from build123d import *

# Parameters (mm, degrees)
F0_W     = 87
F0_H     = 2
F0_W_2   = 29
F1_DEPTH = 2


# Not quite as in the source:
# - ends of sketch curves that miss each other by under 0.0002 mm in the source are joined


with BuildPart() as f1:
    # F0 (on Front) → F1 (new body)
    with BuildSketch(Plane.XZ):
        Polygon((-74.1755201817, -53.7046223087), (-74.1755201817, -54.8843706005), (16.8244798183, -54.8843706005), (16.8244798183, -52.8843706005), (-12.1755201817, -52.8843706005), (-12.1755201817, -50.8843706005), (16.8244798183, -50.8843706005), (16.8244798183, -44.8844749875), (-12.1755201817, -44.8844749875), (-12.1755201817, -42.8844749875), (16.8244798183, -42.8844749875), (16.8244798183, -36.7078750432), (-12.1755201817, -36.7078750432), (-12.1754285991, -34.7078750432), (16.8244798183, -34.7078750432), (16.8244798183, -28.7078750432), (-12.1755201817, -28.7078750432), (-12.1754285991, -26.7078750432), (16.8244798183, -26.7078750432), (16.8244798183, -20.5312750988), (-12.1755201817, -20.5312750988), (-12.1755201817, -18.5312750988), (16.8244798183, -18.5312750988), (16.8244798183, -12.5313794858), (-12.1755201817, -12.5313794858), (-12.1755201817, -10.5313794858), (16.8244798183, -10.5313794858), (16.8244798183, -4.5313794858), (-12.1755201817, -4.5313794858), (-12.1755201817, -2.5313794858), (16.8244798183, -2.5313794858), (16.8244798183, 3.4685161272), (-12.1755201817, 3.4685161272), (-12.1755201817, 5.4685161272), (16.8244798183, 5.4685161272), (16.8244798183, 11.6451160715), (-12.1755201817, 11.6451160715), (-12.1754285991, 13.6451160715), (16.8244798183, 13.6451160715), (16.8244798183, 19.6451160715), (-12.1755201817, 19.6451160715), (-12.1754285991, 21.6451160715), (16.8244798183, 21.6451160715), (16.8244798183, 27.8217160159), (-12.1755201817, 27.8217160159), (-12.1755201817, 29.8217160159), (16.8244798183, 29.8217160159), (16.8244798183, 35.8216116289), (-12.1755201817, 35.8216116289), (-12.1755201817, 37.8216116289), (16.8244798183, 37.8216116289), (16.8244798183, 43.3868200481), (-74.1755201817, 43.3868200481), (-74.1755201817, 37.8216116289), (-45.1755201817, 37.8216116289), (-45.1755201817, 35.8216116289), (-74.1755201817, 35.8216116289), (-74.1755201817, 29.8217160159), (-45.1755201817, 29.8217160159), (-45.1755201817, 27.8217160159), (-74.1755201817, 27.8217160159), (-74.1755201817, 21.6451160715), (-45.1755201817, 21.6451160715), (-45.1754285991, 19.6451160715), (-74.1755201817, 19.6451160715), (-74.1755201817, 13.6451160715), (-45.1755201817, 13.6451160715), (-45.1754285991, 11.6451160715), (-74.1755201817, 11.6451160715), (-74.1755201817, 5.4685161272), (-45.1755201817, 5.4685161272), (-45.1755201817, 3.4685161272), (-74.1755201817, 3.4685161272), (-74.1755201817, -2.5313794858), (-45.1755201817, -2.5313794858), (-45.1755201817, -4.5313794858), (-74.1755201817, -4.5313794858), (-74.1755201817, -10.5313794858), (-45.1755201817, -10.5313794858), (-45.1755201817, -12.5313794858), (-74.1755201817, -12.5313794858), (-74.1755201817, -18.5312750988), (-45.1755201817, -18.5312750988), (-45.1755201817, -20.5312750988), (-74.1755201817, -20.5312750988), (-74.1755201817, -26.7078750432), (-45.1755201817, -26.7078750432), (-45.1754285991, -28.7078750432), (-74.1755201817, -28.7078750432), (-74.1755201817, -34.7078750432), (-45.1755201817, -34.7078750432), (-45.1754285991, -36.7078750432), (-74.1755201817, -36.7078750432), (-74.1755201817, -42.8844749875), (-45.1755201817, -42.8844749875), (-45.1755201817, -44.8844749875), (-74.1755201817, -44.8844749875), (-74.1755201817, -50.8843706005), (-45.1755201817, -50.8843706005), (-45.1755201817, -52.8843706005), (-74.1755201817, -52.8843706005), align=None)
        with Locations((-28.6755201817, -47.8843706005)):
            Rectangle(F0_W, F0_H, mode=Mode.SUBTRACT)
        with Locations((-28.6755201817, -43.8844749875)):
            Rectangle(F0_W_2, F0_H, mode=Mode.SUBTRACT)
        with Locations((-28.6755201817, -31.7078686953)):
            Rectangle(F0_W, F0_H, mode=Mode.SUBTRACT)
        with Locations((-28.6755201817, -19.5312750988)):
            Rectangle(F0_W_2, F0_H, mode=Mode.SUBTRACT)
        with Locations((-28.6755201817, -15.5313794858)):
            Rectangle(F0_W, F0_H, mode=Mode.SUBTRACT)
        with Locations((-28.6755201817, -51.8843706005)):
            Rectangle(F0_W_2, F0_H, mode=Mode.SUBTRACT)
        with Locations((-28.6754285991, -39.7078750432)):
            Rectangle(F0_W, F0_H, mode=Mode.SUBTRACT)
        with Locations((-28.6754285991, -35.7078750432)):
            Rectangle(F0_W_2, F0_H, mode=Mode.SUBTRACT)
        with Locations((-28.6754285991, -27.7078750432)):
            Rectangle(F0_W_2, F0_H, mode=Mode.SUBTRACT)
        with Locations((-28.6754285991, -23.7078750432)):
            Rectangle(F0_W, F0_H, mode=Mode.SUBTRACT)
        with Locations((-28.6755201817, -11.5313794858)):
            Rectangle(F0_W_2, F0_H, mode=Mode.SUBTRACT)
        with Locations((-28.6755201817, -7.5313794858)):
            Rectangle(F0_W, F0_H, mode=Mode.SUBTRACT)
        with Locations((-28.6755201817, 0.4686205142)):
            Rectangle(F0_W, F0_H, mode=Mode.SUBTRACT)
        with Locations((-28.6755201817, 4.4685161272)):
            Rectangle(F0_W_2, F0_H, mode=Mode.SUBTRACT)
        with Locations((-28.6755201817, 16.6451224194)):
            Rectangle(F0_W, F0_H, mode=Mode.SUBTRACT)
        with Locations((-28.6755201817, 28.8217160159)):
            Rectangle(F0_W_2, F0_H, mode=Mode.SUBTRACT)
        with Locations((-28.6755201817, 32.8216116289)):
            Rectangle(F0_W, F0_H, mode=Mode.SUBTRACT)
        with Locations((-28.6755201817, 40.3868200481)):
            Rectangle(F0_W, F0_H, mode=Mode.SUBTRACT)
        with Locations((-28.6755201817, -3.5313794858)):
            Rectangle(F0_W_2, F0_H, mode=Mode.SUBTRACT)
        with Locations((-28.6754285991, 8.6451160715)):
            Rectangle(F0_W, F0_H, mode=Mode.SUBTRACT)
        with Locations((-28.6754285991, 12.6451160715)):
            Rectangle(F0_W_2, F0_H, mode=Mode.SUBTRACT)
        with Locations((-28.6754285991, 20.6451160715)):
            Rectangle(F0_W_2, F0_H, mode=Mode.SUBTRACT)
        with Locations((-28.6754285991, 24.6451160715)):
            Rectangle(F0_W, F0_H, mode=Mode.SUBTRACT)
        with Locations((-28.6755201817, 36.8216116289)):
            Rectangle(F0_W_2, F0_H, mode=Mode.SUBTRACT)
    extrude(amount=F1_DEPTH)


solid = f1.part
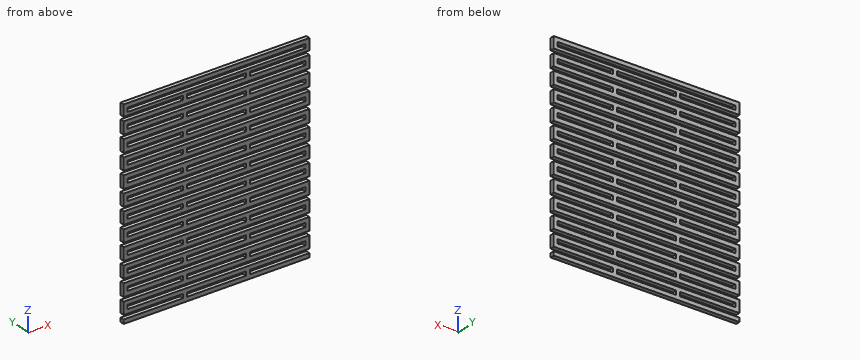
Verification items for the finished model (mm, model axes). Coordinates: 2 decimals unless noted, no trailing zeros.
1. Go/stop test with flat-tipped pins: pin 1 Ø0.6 at (y, z) = (-1, -3) entering from +X; pin 2 Ø1.5 at (x, z) = (-59, -24) entering from -Y. Record where each tip stops, or that it passes through.
Results found:
pin 1: stops at x = -12.18
pin 2: stops at y = -2
2. Sectioned sample at A-A, the plane x = -37.5. Give the number of separate pieces and of enclosed holes in the cut face, and give its area (3 significant figures).
Results found:
separate pieces: 25
enclosed holes: 0
area: 101 mm2
3. Scan lines: line 1 (X direction, y = -0.6, z = 0.5); line 2 (X direction, y = -0.4, z = 5). Record each from-to range of solid material in increasing order.
Results found:
line 1: x = -74.18 to -72.18, 14.82 to 16.82
line 2: x = -45.18 to -43.18, -14.18 to -12.18
